```python
from build123d import *

# Parameters (mm, degrees)
SKETCH1_R           = 1.55
BOSS_EXTRUDE1_DEPTH = 5
SKETCH2_W           = 25.9
SKETCH2_H           = 28.1
SKETCH2_W_2         = 22.9
SKETCH2_H_2         = 25.1
BOSS_EXTRUDE2_DEPTH = 15.7
CUT_EXTRUDE1_DEPTH  = 2


with BuildPart() as part:
    # Sketch1 → Boss-Extrude1 (new body)
    with BuildSketch(Plane(origin=(0, 0, 0), x_dir=(1, 0, 0), z_dir=(0, 1, 0))):
        Polygon((0, 25.1), (-3, 25.1), (-3, -3), (22.9, -3), (22.9, 25.1), align=None)
        with Locations(Location((17.36, 2.54, 0), (0, 0, 270))):
            Circle(SKETCH1_R, mode=Mode.SUBTRACT)
        with Locations(Location((4.76, 19.54, 0), (0, 0, 270))):
            Circle(SKETCH1_R, mode=Mode.SUBTRACT)
    extrude(amount=BOSS_EXTRUDE1_DEPTH)

    # Sketch2 → Boss-Extrude2 (add)
    with BuildSketch(Plane(origin=(0, 5, 0), x_dir=(1, 0, 0), z_dir=(0, 1, 0))):
        with Locations((9.95, 11.05)):
            Rectangle(SKETCH2_W, SKETCH2_H)
        with Locations((9.95, 11.05)):
            Rectangle(SKETCH2_W_2, SKETCH2_H_2, mode=Mode.SUBTRACT)
    extrude(amount=BOSS_EXTRUDE2_DEPTH)

    # Sketch3 → Cut-Extrude1 (cut)
    with BuildSketch(Plane.ZY.offset(3)):
        Polygon((-11.05, 4.5), (-20.05, 4.5), (-20.05, 5.75), (-2.05, 5.75), (-2.05, 4.5), align=None)
    extrude(amount=-CUT_EXTRUDE1_DEPTH, mode=Mode.SUBTRACT)


solid = part.part
```
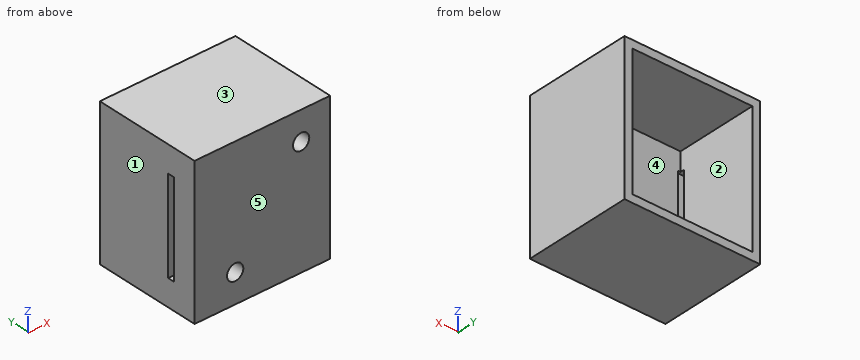
Geometry: final body of the model. Coordinates: model frame, mm. Face numbers are marked on the shaded views. A direction names the side the tool comes from. Coordinates: 2 decimals unless noted, no trailing zeros. Order: outer loops, then holes, each group sorted by start corner. A loop starts at its lowest first (then second) coordinate and runs counter-clockwise, first axis right, second up. Notation, with made-up numbers: (75, 48) - (126, 48) arc R16 cw to (126, 58) - close; hole circle Ø4 at (7, 47). An arc over 180 degrees is marked (long way). Write each question's results on one line, items separated by ' | '.
(1) Section query A-A, the plane z = -19.54. Return the cut outline in (x, y), plus the area to 3 significant figures.
Values found:
outline: (-3, 0) - (3.21, 0) - (3.21, 5) - (-1, 5) - (-1, 4.5) - (-3, 4.5) - close; (-3, 5.75) - (-1.5, 5.75) - (-1.5, 20.7) - (-3, 20.7) - close; (6.31, 0) - (22.9, 0) - (22.9, 20.7) - (21.4, 20.7) - (21.4, 5) - (6.31, 5) - close | area: 159 mm²
(2) Section query D-D, the plane z = -5. Return the cut outline in (x, y), plus the area to 3 significant figures.
Values found:
outline: (-3, 0) - (22.9, 0) - (22.9, 20.7) - (21.4, 20.7) - (21.4, 5) - (-1, 5) - (-1, 4.5) - (-3, 4.5) - close; (-3, 5.75) - (-1.5, 5.75) - (-1.5, 20.7) - (-3, 20.7) - close | area: 174 mm²
(3) Section query B-B, the plane x = 17.36. Return the cut outline in (y, z).
Values found:
outline: (0, -25.1) - (20.7, -25.1) - (20.7, -23.6) - (5, -23.6) - (5, -4.09) - (0, -4.09) - close; (0, -0.99) - (5, -0.99) - (5, 1.5) - (20.7, 1.5) - (20.7, 3) - (0, 3) - close
(4) First-contact query: pin 1 Ø2.5 at (x, z) = (4.76, -19.54) entering from +Y; pin 2 Ø5 at (x, z) = (12, -19) entering from +Y. Flat tips, straight axial feed; report the tip coordinate or a pass-through.
Values found:
pin 1: passes through | pin 2: stops at y = 5
(5) Section query C-C, the plane y = 19. Return the cut outline in (x, z).
Values found:
outline: (-3, -25.1) - (22.9, -25.1) - (22.9, 3) - (-3, 3) - close; hole (-1.5, -23.6) - (21.4, -23.6) - (21.4, 1.5) - (-1.5, 1.5) - close
(6) Line query: line 1 (Z direction, x = 19, y = 12.5); line 2 (X direction, y = 1.15, z = -2.54); line 3 (X direction, y = 19.5, z = -11.5). Output: solid intervals per line, ascending. Write a range as [from, to].
Values found:
line 1: z = [-25.1, -23.6], [1.5, 3] | line 2: x = [-3, 15.81], [18.91, 22.9] | line 3: x = [-3, -1.5], [21.4, 22.9]
(7) Set-up query: the marked faces 4 and 5. Return all of +Z, -Z, +X, -X, +Y, -Y with unobstructed straight access to the full face (end or side cutting, diameter ignored); none if empty.
Values found:
face 4: +Y | face 5: +Z, -Z, +X, -X, -Y
(8) Mould query, pull axis X, two halves, no side actions, for the marked faces 1, 2 and 3. Classes: +X half, -X half, draft (parallel to the pull), parting line (faces both ways), or undercut.
Values found:
face 1: -X half | face 2: undercut | face 3: draft
